Geometry: final body of the model. Coordinates: model frame, mm. A direction names the side the tool comes from. Coordinates: 2 decimals unless noted, no trailing zeros. Order: outer loops, then holes, each group sorted by start corner. A loop starts at its lowest first (then second) coordinate and runs counter-clockwise, first axis right, second up. Notation, with made-up numbers: (38.25, 66.5) -> (94.25, 66.5) arc R26 cw to (94.25, 86.5) -> close; hole circle Ø6 at (-8, 66). An arc over 180 degrees is marked (long way). Use CSV: the item, a comma, the result in double quotes. Start each with the question number.
Autodesk Inventor part; units mm, degrees
ref_plane "YZ Plane" through (0, 0, 0) normal (1, 0, 0) x (0, 1, 0)
ref_plane "XZ Plane" through (0, 0, 0) normal (0, 1, 0) x (-1, 0, 0)
ref_plane "XY Plane" through (0, 0, 0) normal (0, 0, 1) x (1, 0, 0)
sketch "스케치1" plane through (0, 0, 0) normal (0, 0, 1) x (1, 0, 0)
  line L0 (-13, -5) -> (13, -5)
  line L1 (13, -5) -> (13, 5)
  line L2 (13, 5) -> (-13, 5)
  line L3 (-13, 5) -> (-13, -5)
  line L4 (-13, -5) -> (13, 5) construction
  line L5 (13, -5) -> (-13, 5) construction
  point P0 (0, 0)
  dimension "d0" = 26
  dimension "d1" = 10
extrude "돌출1" add sketch "스케치1" along normal blind 15
sketch "스케치2" plane through (-13, -5, 0) normal (0, -1, 0) x (1, 0, 0)
  circle A0 centre (13, 2.5) radius 1.5
  line L0 (0, 0) -> (26, 0)
  line L1 (0, 0) -> (0, 15)
  circle A1 centre (23.5, 2.5) radius 1.5
  line L2 (26, 0) -> (26, 15)
  point P0 (13, 0)
  point P1 (13, 0)
  point P2 (13, 0)
  dimension "d4" = 3
  dimension "d7" = 2.5
  dimension "d11" = 2.5
  dimension "d12" = 2.5
extrude "돌출2" cut sketch "스케치2" against normal through all
sketch "스케치3" plane through (0, 0, 15) normal (0, 0, 1) x (1, 0, 0)
  circle A0 centre (0, 0) radius 2.5
  dimension "d8" = 5
extrude "돌출3" cut sketch "스케치3" against normal blind 5
sketch "스케치5" plane through (-13, 5, 0) normal (0, 1, 0) x (1, 0, 0)
  line L0 (26, -15) -> (34.5549, -15)
  line L1 (34.5549, -15) -> (56, -5)
  line L2 (56, -5) -> (56, 0)
  line L3 (56, 0) -> (26, 0)
  circle A0 centre (53.5, -2.5) radius 1.5
  line L4 (26, 0) -> (26, -15)
  point P0 (13, 0)
  point P1 (56, -2.5)
  dimension "d13" = 5
  dimension "d14" = 115
  dimension "d15" = 30
  dimension "d16" = 3
  dimension "d17" = 2.5
extrude "돌출4" add sketch "스케치5" against normal up to surface (10 mm away)
equation "\"d11\" = d7"
equation "\"d12\" = d11"
properties part number "Steering"
(1) Section D-D (z = 13.75). Return loops of the section in (x, y).
(2) First-contact query: pin 1 (1.5 mm diameter, centred on x = 0.5, y = -0.5, fed in from +Z). Flat tip, straight axial feed; report the tip coordinate or a pass-through.
(3) Line query: line 1 (Y direction, x = 0, z = 12.8); line 2 (X direction, y = -1.75, z = 3); line 3 (Z direction, x = 0, y = 3.25). Output: solid intervals per line, ascending. Write a range as from..to.
(4) Section C-C (y = 2). Return loops of the section in (x, z).
(5) Access query for faces 1 (the face through (-0.54, -2.44, 12.54)), 2 (the face through (15, 5, 7)). Directions: +Z, -Z, +X, -X, +Y, -Y. A direction counts if a zero-diameter tool reaches every point of the face in a straight line with its end or side. Return the directions, or none.
(6) Section B-B (x = 0). Return loops of the section in (y, z).
(7) Section A-A (z = 2.5). Return loops of the section in (x, y), then the cut area to 3 significant figures.
(8) Mould query, pull axis Z, two halves, no side actions, for faces 3 (the face through (0, 0, 1)), 4 (the face through (0, 0, 10)), 5 (the face through (15, 0, 0)). Classes: pulls with the +Z half, pulls with the -Z half, needs draft (parallel to the pull), parting line crosses it, or undercut.
Check sheet entries:
1,outline,"(-13, -5) -> (24.24, -5) -> (24.24, 5) -> (-13, 5) -> close; hole circle Ø5 at (0, 0)"
2,pin 1,"stops at z = 10"
3,line 1,"y = -5..-2.5, 2.5..5"
3,line 2,"x = -13..-1.41, 1.41..9.09, 11.91..39.09, 41.91..43"
3,line 3,"z = 0..1, 4..15"
4,outline,"(-13, 0) -> (43, 0) -> (43, 5) -> (21.55, 15) -> (1.5, 15) -> (1.5, 10) -> (-1.5, 10) -> (-1.5, 15) -> (-13, 15) -> close; hole circle Ø3 at (0, 2.5); hole circle Ø3 at (10.5, 2.5); hole circle Ø3 at (40.5, 2.5)"
5,face 1,"+Z"
5,face 2,"+Z, -Z, +X, -X, +Y"
6,outline,"(-5, 0) -> (5, 0) -> (5, 1) -> (-5, 1) -> close; (-5, 4) -> (5, 4) -> (5, 15) -> (2.5, 15) -> (2.5, 10) -> (-2.5, 10) -> (-2.5, 15) -> (-5, 15) -> close"
7,outline,"(-13, -5) -> (-1.5, -5) -> (-1.5, 5) -> (-13, 5) -> close; (1.5, -5) -> (9, -5) -> (9, 5) -> (1.5, 5) -> close; (12, -5) -> (39, -5) -> (39, 5) -> (12, 5) -> close; (42, -5) -> (43, -5) -> (43, 5) -> (42, 5) -> close"
7,area,"470 mm^2"
8,face 3,"undercut"
8,face 4,"pulls with the +Z half"
8,face 5,"pulls with the -Z half"
